Autodesk Inventor part; units mm, degrees
ref_plane "YZ Plane" through (0, 0, 0) normal (1, 0, 0) x (0, 1, 0)
ref_plane "XZ Plane" through (0, 0, 0) normal (0, 1, 0) x (-1, 0, 0)
ref_plane "XY Plane" through (0, 0, 0) normal (0, 0, 1) x (1, 0, 0)
sketch "Sketch1" plane through (0, 0, 0) normal (0, 0, 1) x (1, 0, 0)
  line L0 (-6.0954, 5.4228) -> (18.9046, 5.4228)
  line L1 (18.9046, 5.4228) -> (18.9046, -19.5772)
  line L2 (18.9046, -19.5772) -> (-6.0954, -19.5772)
  line L3 (-6.0954, -19.5772) -> (-6.0954, 5.4228)
  line L4 (-6.0954, -22.5772) -> (21.9046, -22.5772)
  line L5 (21.9046, -22.5772) -> (21.9046, 5.4228)
  line L6 (18.9046, 5.4228) -> (21.9046, 5.4228)
  line L7 (-6.0954, -19.5772) -> (-6.0954, -22.5772)
  point P0 (0, 0)
  point P1 (6.4046, -7.0772)
  dimension "d0" = 25
  dimension "d1" = 25
  dimension "d2" = 3
  dimension "d3" = 3
  dimension "d4" = 12.5
  dimension "d5" = 12.5
extrude "Extrusion1" add sketch "Sketch1" along normal blind 6
extrude "Extrusion2" add sketch "Sketch1" against normal blind 2 contours L6 L5 L4 L7 L2 L1
hole "Hole1" at (6.4046, -7.0772, 0) direction (0, 0, 1) diameter 4 end through all
sketch "Sketch2" plane through (0, 0, 6) normal (0, 0, 1) x (1, 0, 0)
  circle A0 centre (6.4046, -7.0772) radius 2
  line L0 (-6.0954, 5.4228) -> (-6.0954, -22.5772)
  line L1 (-6.0954, -22.5772) -> (21.9046, -22.5772)
  line L2 (21.9046, -22.5772) -> (21.9046, 5.4228)
  line L3 (21.9046, 5.4228) -> (-6.0954, 5.4228)
  circle A1 centre (6.4046, -7.0772) radius 2
  circle A2 centre (6.4046, -7.0772) radius 4.5
  point P0 (0, 0)
  dimension "d17" = 9
extrude "Extrusion3" cut sketch "Sketch2" against normal blind 1.5 contours A2
chamfer "Chamfer1" distance 2 angle 45 1 edges at (6.4046, -9.0772, 4.5)
fillet "Fillet1" radius 2 2 edges at (21.9046, -22.5772, 2) (-6.0954, 5.4228, 3)
properties part number "3DP_PLA_Base_plate_corner_leg" material "ABS Plastic"
Input: part model. Units: mm. Frame: model coordinates. A direction names the side the tool comes from. Give positions to 0.01 mm unless a question says otherwise; leave off trailing zeros. Order: outer loops, then holes, each group sorted by start corner. A loop starts at its lowest first (then second) coordinate and runs counter-clockwise, first axis right, second up. Notation, with made-up numbers: (23, 12) - (29, 12) arc R21 cw to (29, 39) - close; hole circle Ø8 at (-30, 15). An arc over 180 degrees is marked (long way). Use a Markdown table: item, result.
(1) Section query A-A (z = 3.5). Output: boundary loops of the cut face in (x, y).
Computed values:
| item | result |
|---|---|
| outline | (-6.1, -22.58) - (19.9, -22.58) arc R2 ccw to (21.9, -20.58) - (21.9, 5.42) - (-4.1, 5.42) arc R2 ccw to (-6.1, 3.42) - close; hole circle Ø6 at (6.4, -7.08) |
(2) Access query for faces 1 (the flat face through (14, -20, -2)), 2 (the cylindrical face through (10.56, -8.8, 5.26)), 3 (the flat face through (18.905, -7, -1)). Directions: +Z, -Z, +X, -X, +Y, -Y. A direction counts if a zero-diameter tool reaches every point of the face in a straight line with its end or side. Return the directions, or none.
Computed values:
| item | result |
|---|---|
| face 1 | -Z, +X, -X, +Y, -Y |
| face 2 | +Z |
| face 3 | -Z, -X, +Y |
(3) Section query C-C (y = -14). Output: boundary loops of the cut face in (x, z).
Computed values:
| item | result |
|---|---|
| outline | (-6.1, 0) - (18.9, 0) - (18.9, -2) - (21.9, -2) - (21.9, 6) - (-6.1, 6) - close |
(4) Section query B-B (x = 17.25). Output: boundary loops of the cut face in (y, z).
Computed values:
| item | result |
|---|---|
| outline | (-22.58, -2) - (-19.58, -2) - (-19.58, 0) - (5.42, 0) - (5.42, 6) - (-22.58, 6) - close |
(5) Section query D-D (z = 0.5). Output: boundary loops of the cut face in (x, y), then the cut area to 3 significant figures.
Computed values:
| item | result |
|---|---|
| outline | (-6.1, -22.58) - (19.9, -22.58) arc R2 ccw to (21.9, -20.58) - (21.9, 5.42) - (-4.1, 5.42) arc R2 ccw to (-6.1, 3.42) - close; hole circle Ø4 at (6.4, -7.08) |
| area | 770 mm2 |
(6) Pin query (flat end, axial travel): pin 1 (2 mm diameter, centred on x = 9, z = -1.5, fed in from +Y); pin 2 (7.5 mm diameter, centred on x = 2.5, y = -11, fed in from -Z); pin 3 (0.6 mm diameter, centred on y = -10, z = -1.5, fed in from -X). Return the tip coordinate at first contact, or that it passes through.
Computed values:
| item | result |
|---|---|
| pin 1 | stops at y = -19.58 |
| pin 2 | stops at z = 0 |
| pin 3 | stops at x = 18.9 |
(7) Line query: line 1 (Z direction, x = -3, y = 1.5); line 2 (Y direction, x = 12, z = -1.5); line 3 (Y direction, x = 3.5, z = 5). Output: solid intervals per line, ascending. Write a range as from..to.
Computed values:
| item | result |
|---|---|
| line 1 | z = 0..6 |
| line 2 | y = -22.58..-19.58 |
| line 3 | y = -22.58..-10.51, -3.64..5.42 |
(8) Draft query along X for faces 4 (the conical face through (4.61, -5.93, 2.63)), 5 (the flat face through (9, 5.423, 3)), 6 (the flat face through (21.905, -8, 2)). Return one class per face: released by +X, released by -X, zero draft, split by the parting line, or undercut.
Computed values:
| item | result |
|---|---|
| face 4 | undercut |
| face 5 | zero draft |
| face 6 | released by +X |
